from build123d import *

# Parameters (mm, degrees)
BOSS_EXTRUDE1_DEPTH = 1700
SKETCH3_R           = 7
CUT_EXTRUDE1_DEPTH  = 10
SKETCH5_R           = 40
CUT_EXTRUDE3_DEPTH  = 30
LPATTERN2_COUNT     = 4
LPATTERN2_PITCH     = 366


with BuildPart() as part:
    # Sketch1 → Boss-Extrude1 (new body)
    with BuildSketch(Plane(origin=(0, 0, 0), x_dir=(0, 0, -1), z_dir=(1, 0, 0))):
        with BuildLine():
            Line((-86.622073579, 113.879598662), (-186.622073579, 113.879598662))
            Line((-186.622073579, 113.879598662), (-186.622073579, -186.120401338))
            Line((-186.622073579, -186.120401338), (-86.622073579, -186.120401338))
            Line((-86.622073579, -186.120401338), (-86.622073579, -180.120401338))
            ThreePointArc((-86.622073579, -180.120401338), (-89.551005767, -173.049333526), (-96.622073579, -170.120401338))
            Line((-96.622073579, -170.120401338), (-166.622073579, -170.120401338))
            ThreePointArc((-166.622073579, -170.120401338), (-173.69314139, -167.19146915), (-176.622073579, -160.120401338))
            Line((-176.622073579, -160.120401338), (-176.622073579, 87.879598662))
            ThreePointArc((-176.622073579, 87.879598662), (-173.69314139, 94.950666474), (-166.622073579, 97.879598662))
            Line((-166.622073579, 97.879598662), (-96.622073579, 97.879598662))
            ThreePointArc((-96.622073579, 97.879598662), (-89.551005767, 100.80853085), (-86.622073579, 107.879598662))
            Line((-86.622073579, 107.879598662), (-86.622073579, 113.879598662))
        make_face()
    extrude(amount=BOSS_EXTRUDE1_DEPTH)

    # Sketch3 → Cut-Extrude1 (cut)
    with BuildSketch(Plane.XY.offset(186.622073579)):
        with Locations((1655, 38.879598662)):
            Circle(SKETCH3_R)
        with Locations((1655, -36.120401338)):
            Circle(SKETCH3_R)
        with Locations((1655, -111.120401338)):
            Circle(SKETCH3_R)
    cut_extrude1 = extrude(amount=-CUT_EXTRUDE1_DEPTH, mode=Mode.SUBTRACT)

    # Mirror1: Cut-Extrude1 across plane
    add(cut_extrude1.mirror(Plane(origin=(850, 0, 0), x_dir=(0, 0, 1), z_dir=(1, 0, 0))), mode=Mode.SUBTRACT)

    # Sketch5 → Cut-Extrude3 (cut)
    with BuildSketch(Plane(origin=(0, 0, 176.622073579), x_dir=(-1, 0, 0), z_dir=(0, 0, -1))):
        with Locations(Location((-1399, -36.120401338, 0), (0, 0, 90))):
            Circle(SKETCH5_R)
    cut_extrude3 = extrude(amount=-CUT_EXTRUDE3_DEPTH, mode=Mode.SUBTRACT)

    # LPattern2: Cut-Extrude3 ×4
    with Locations(*[(-i * LPATTERN2_PITCH, 0, 0) for i in range(1, LPATTERN2_COUNT)]):
        add(cut_extrude3, mode=Mode.SUBTRACT)


solid = part.part
Work out the finished part from the listing and answer in its coordinate system (mm). A direction names the side the tool comes from. Give positions to 0.01 mm unless a question says otherwise; leave off trailing zeros. Write each loop counter-clockwise with the first axis right and the second up, starting at its lowest first coordinate (ties: lowest second). Pieces come first, ordered by that corner, then holes.
Q1. Straight lines are drawn through the part: L1, parallel to Y at x = 1655, z = 182; L2, parallel to Y at x = 1285.5, z = 139.5; L3, parallel to Z at x = 1606, y = 87. For each, find the intervals that lie inside material, in ascending order.
Answer:
L1: y = -186.12 to -118.12, -104.12 to -43.12, -29.12 to 31.88, 45.88 to 113.88
L2: y = -186.12 to -170.12, 97.88 to 113.88
L3: z = 176.62 to 186.62
Q2. For a pull along Y with two mould halves and no side action, classify faces 1 (the face through (838, 113.88, 136)), 2 (the face through (838, -38, 176.622)), 3 (the face through (1700, -13, 178)) as released by +Y, released by -Y, zero draft, split by the parting line, or undercut.
Answer:
face 1: released by +Y
face 2: undercut
face 3: zero draft
Q3. Given pin 1 (1.5 mm diameter, centred on y = -101, z = 176.5, fed in from +X); pin 2 (16 mm diameter, centred on x = 45, y = 38.88, fed in from -Z), each flat-ended and moving along its own axis, determine where each tip first touches the part or whether it passes through.
Answer:
pin 1: stops at x = 1700
pin 2: stops at z = 176.62
Q4. The part is cut by section B-B on x = 301. Give the vertices of the cut face in (y, z), and give its area (3 significant figures).
Answer:
outline: (-186.12, 86.62) - (-180.12, 86.62) arc R10 ccw to (-170.12, 96.62) - (-170.12, 166.62) arc R10 cw to (-160.12, 176.62) - (-76.12, 176.62) - (-76.12, 186.62) - (-186.12, 186.62) - close; (3.88, 176.62) - (87.88, 176.62) arc R10 cw to (97.88, 166.62) - (97.88, 96.62) arc R10 ccw to (107.88, 86.62) - (113.88, 86.62) - (113.88, 186.62) - (3.88, 186.62) - close
area: 5,080 mm2
Q5. The part is cut by section C-C on y = -134. Give the vertices of the cut face in (x, z), and give its area (3 significant figures).
Answer:
outline: (0, 176.62) - (1700, 176.62) - (1700, 186.62) - (0, 186.62) - close
area: 17,000 mm2
Q6. A tool of negligible diameter and unlimited length cuts with its end or side. For faces 4 (the face through (340.66, -41.33, 181.55)), 5 (the face through (838, 97.88, 132)), from which of +Z, -Z, +X, -X, +Y, -Y can it reach the whole face along a straight path? Write none if from no direction.
Answer:
face 4: +Z, -Z
face 5: -Z, +X, -X
Q7. The part is cut by section A-A on z = 120. Give the vertices of the cut face in (x, y).
Answer:
outline: (0, -186.12) - (1700, -186.12) - (1700, -170.12) - (0, -170.12) - close; (0, 97.88) - (1700, 97.88) - (1700, 113.88) - (0, 113.88) - close
